Could you check a few things on this drawing? It's one solid part, dimensions in mm from its lowest x, y, z. A direction names the side the tool comes from. Round coordinates to 2 decimals unless told otherwise and drop trailing zeros. Loops run counter-clockwise (first coordinate to the right, second up) from the corner with the lowest first, then second, coordinate; pieces in that order, holes last. Notation, with made-up numbers: (44.5, -16) -> (54.5, -16) arc R23 ccw to (54.5, 12) -> close; hole circle Ø3 at (-23.75, 10.5). An arc over 180 degrees is marked (long way). Use one line per item in the form item = value. Start each with the question number.
Item 1: If we section it at C-C (z = 33): Write out the boundary of the cut face in (x, y), then the cut area to 4 significant figures.
Item 2: If we section it at B-B (y = 26.5): Write out the boundary of the cut face in (x, z), then the cut area to 3 significant figures.
Item 3: I'm going to push flat-ended pins straight in: pin 1 Ø5 at (y, z) = (22.5, 15) entering from -X; pin 2 Ø2 at (y, z) = (36.5, 14.5) entering from +X; pin 3 Ø2.5 at (x, y) = (53, 29.5) entering from -Z; pin 4 Ø8 at (x, y) = (33, 8.5) entering from -Z. Where does each tip first touch, or does it pass through?
Item 4: If we section it at A-A (y = 20.5): Write out the boundary of the cut face in (x, z), then the cut area to 3 significant figures.
Item 5: For the marked faces 1, 2 and 3, which set-ups out of +Z, -Z, +X, -X, +Y, -Y let a thin tool reach every point of the face, with its end or its side?
Item 6: If I drill on L1, parallel to X at y = 3, z = 34.75; L2, parallel to Y at x = 3, z = 34.7; L3, parallel to Y at x = 53, z = 35 (1 decimal), over which ranges is the centre line in solid material (lowest first)? Write a range as [from, to].
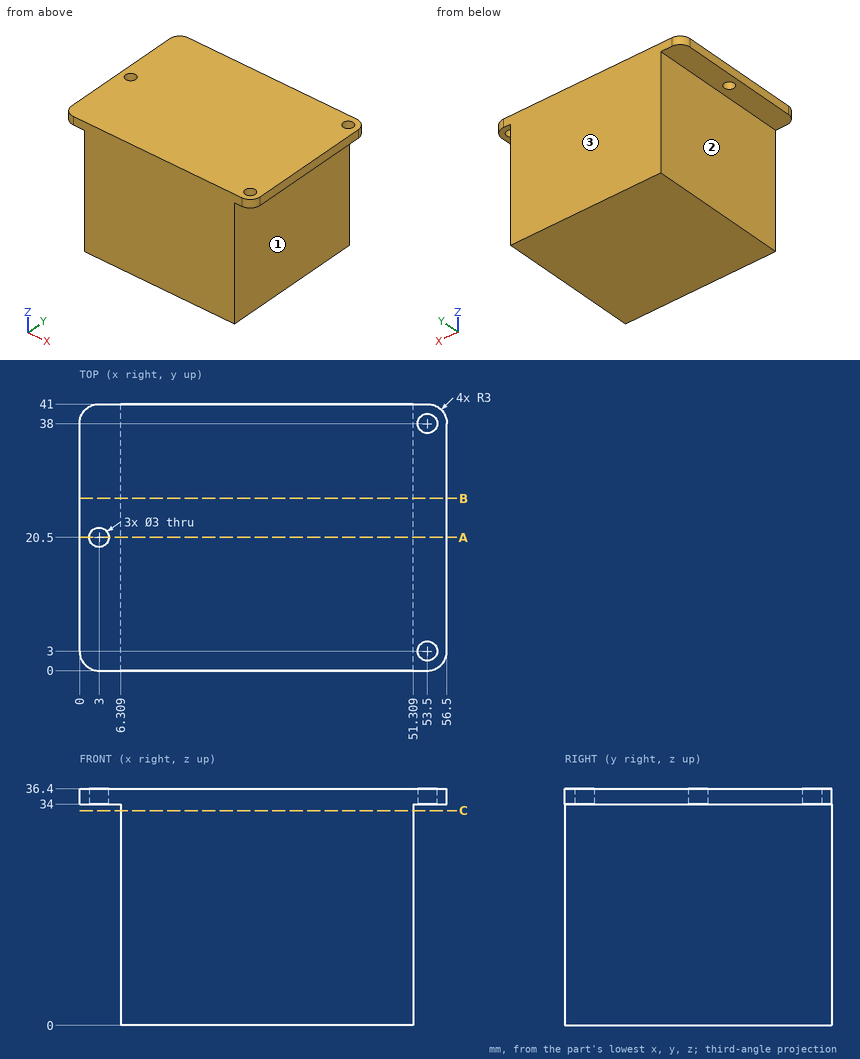
Values found:
q1.outline = (6.31, 0) -> (51.31, 0) -> (51.31, 41) -> (6.31, 41) -> close
q1.area = 1,845 mm2
q2.outline = (0, 34) -> (6.31, 34) -> (6.31, 0) -> (51.31, 0) -> (51.31, 34) -> (56.5, 34) -> (56.5, 36.4) -> (0, 36.4) -> close
q2.area = 1,670 mm2
q3.pin_1 = 6.31
q3.pin_2 = 51.31
q3.pin_3 = 34
q3.pin_4 = 0
q4.outline = (0, 34) -> (1.5, 34) -> (1.5, 36.4) -> (0, 36.4) -> close; (4.5, 34) -> (6.31, 34) -> (6.31, 0) -> (51.31, 0) -> (51.31, 34) -> (56.5, 34) -> (56.5, 36.4) -> (4.5, 36.4) -> close
q4.area = 1,660 mm2
q5.face_1 = -Z, +X, +Y, -Y
q5.face_2 = -Z, -X, +Y, -Y
q5.face_3 = +Z, -Z, +X, -X, +Y
q6.L1 = [0, 52], [55, 56.5]
q6.L2 = [0, 19], [22, 41]
q6.L3 = [0, 1.6], [4.4, 36.6], [39.4, 41]
